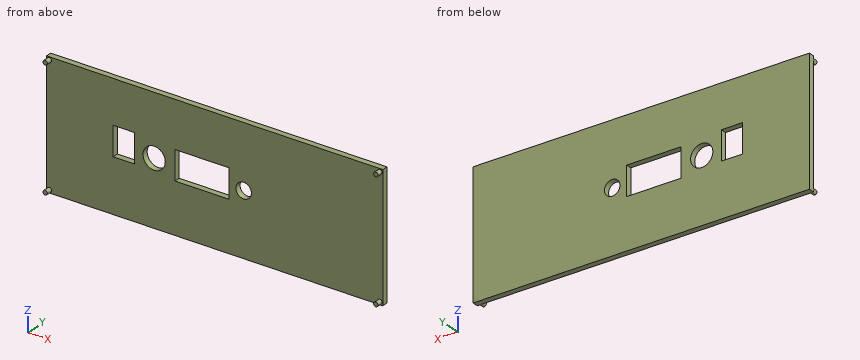
```python
from build123d import *

# Parameters (mm, degrees)
SKETCH1_W           = 174
SKETCH1_H           = 65
BOSS_EXTRUDE1_DEPTH = 3
SKETCH2_R           = 4
SKETCH2_R_2         = 5.75
SKETCH2_W           = 28
SKETCH2_H           = 15
SKETCH2_W_2         = 11
CUT_EXTRUDE1_DEPTH  = 3
SKETCH3_R           = 1.15
BOSS_EXTRUDE2_DEPTH = 3


with BuildPart() as part:
    # Sketch1 → Boss-Extrude1 (new body)
    with BuildSketch(Plane(origin=(0, 0, 0), x_dir=(1, 0, 0), z_dir=(0, 1, 0))):
        Rectangle(SKETCH1_W, SKETCH1_H)
    extrude(amount=BOSS_EXTRUDE1_DEPTH)

    # Sketch2 → Cut-Extrude1 (cut)
    with BuildSketch(Plane(origin=(0, 3, 0), x_dir=(1, 0, 0), z_dir=(0, 1, 0))):
        with Locations(Location((15, 0, 0), (0, 0, 270))):
            Circle(SKETCH2_R)
        with Locations(Location((-31.3, -1.00957594, 0), (0, 0, 270))):
            Circle(SKETCH2_R_2)
        with Locations((-6.5, -1.00957594)):
            Rectangle(SKETCH2_W, SKETCH2_H)
        with Locations((-47, -2.596032883)):
            Rectangle(SKETCH2_W_2, SKETCH2_H)
    extrude(amount=-CUT_EXTRUDE1_DEPTH, mode=Mode.SUBTRACT)

    # Sketch3 → Boss-Extrude2 (add)
    with BuildSketch(Plane.XZ):
        with Locations(Location((-85.5, 31, 0), (0, 0, 270))):
            Circle(SKETCH3_R)
        with Locations(Location((85.5, 31, 0), (0, 0, 270))):
            Circle(SKETCH3_R)
        with Locations(Location((85.5, -31, 0), (0, 0, 270))):
            Circle(SKETCH3_R)
        with Locations(Location((-85.5, -31, 0), (0, 0, 270))):
            Circle(SKETCH3_R)
    extrude(amount=BOSS_EXTRUDE2_DEPTH)


solid = part.part
```
Can you work these out from the model? Positions are in its coordinate system, mm. Give positions to 0.01 mm unless a question says otherwise; leave off trailing zeros. Order: outer loops, then holes, each group sorted by start corner. A loop starts at its lowest first (then second) coordinate and runs counter-clockwise, first axis right, second up. Notation, with made-up numbers: (-22, 83.25) - (-4, 83.25) arc R25 ccw to (-4, 121.25) - close; hole circle Ø8 at (32.25, 24). An arc over 180 degrees is marked (long way). Use a Markdown table: item, result. Add a question column.
Q1. Please list where these lines run through material, in increasing order: line 1 along X through (y, z) = (0.5, 8); line 2 along Z through (x, y) = (2.5, 2.05); line 3 along X through (y, z) = (1.45, 6).
Q2. If we section it at A-A on x = 15: Write out the boundary of the cut face in (y, z).
Q3. If we section it at C-C on x = -13.5: Write out the boundary of the cut face in (y, z), plus the area to 3 significant figures.
Q4. I'm going to push a flat-ended pin straight in: pin 1 (13 mm diameter, centred on x = -31.3, z = 1.01, fed in from -Y). Where does the tip first touch, or does it pass through?
Q5. If we section it at D-D on z = 15: Write out the boundary of the cut face in (x, y), plus the area to 3 significant figures.
Q6. If we section it at B-B on z = 0: Write out the boundary of the cut face in (x, y).
Answers follow:
| question | item | result |
|---|---|---|
| 1 | line 1 | x = -87 to -52.5, -41.5 to -20.5, 7.5 to 87 |
| 1 | line 2 | z = -32.5 to -6.49, 8.51 to 32.5 |
| 1 | line 3 | x = -87 to -52.5, -41.5 to -34.16, -28.44 to -20.5, 7.5 to 87 |
| 2 | outline | (0, -32.5) - (3, -32.5) - (3, -4) - (0, -4) - close; (0, 4) - (3, 4) - (3, 32.5) - (0, 32.5) - close |
| 3 | outline | (0, -32.5) - (3, -32.5) - (3, -6.49) - (0, -6.49) - close; (0, 8.51) - (3, 8.51) - (3, 32.5) - (0, 32.5) - close |
| 3 | area | 150 mm^2 |
| 4 | pin 1 | stops at y = 0 |
| 5 | outline | (-87, 0) - (87, 0) - (87, 3) - (-87, 3) - close |
| 5 | area | 522 mm^2 |
| 6 | outline | (-87, 0) - (-52.5, 0) - (-52.5, 3) - (-87, 3) - close; (-41.5, 0) - (-36.96, 0) - (-36.96, 3) - (-41.5, 3) - close; (-25.64, 0) - (-20.5, 0) - (-20.5, 3) - (-25.64, 3) - close; (7.5, 0) - (11, 0) - (11, 3) - (7.5, 3) - close; (19, 0) - (87, 0) - (87, 3) - (19, 3) - close |
